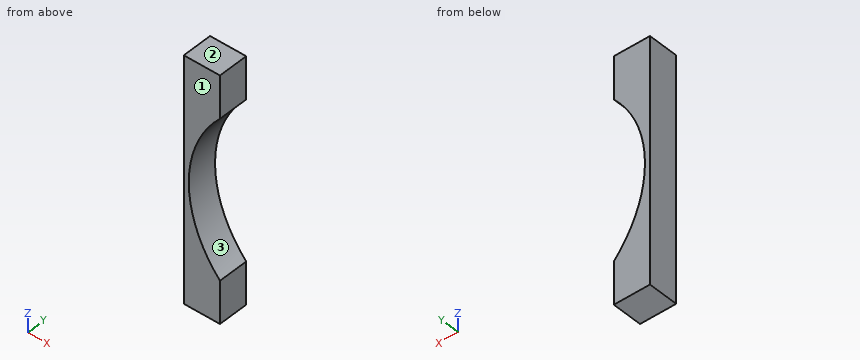
```python
from build123d import *

# Parameters (mm, degrees)
SKETCH1_W           = 24.21
SKETCH1_H           = 6
BOSS_EXTRUDE1_DEPTH = 48.61
CUT_EXTRUDE1_DEPTH  = 53.417790043


with BuildPart() as part:
    # Sketch1 → Boss-Extrude1 (new body)
    with BuildSketch(Plane.XY):
        with Locations((-6.568312856, 6.986625)):
            Rectangle(SKETCH1_W, SKETCH1_H)
    extrude(amount=BOSS_EXTRUDE1_DEPTH)

    # Sketch3 → Cut-Extrude1 (cut, through all)
    with BuildSketch(Plane(origin=(0, 9.986625, 0), x_dir=(1, 0, 0), z_dir=(0, 1, 0))):
        with BuildLine():
            Line((-11.463312856, 0), (-11.463312856, -8.458721642))
            ThreePointArc((-11.463312856, -8.458721642), (-17.673312856, -24.3), (-11.463312856, -40.141278358))
            Line((-11.463312856, -40.141278358), (-11.463312856, -48.61))
            Line((-11.463312856, -48.61), (5.536687144, -48.61))
            Line((5.536687144, -48.61), (5.536687144, 0))
            Line((5.536687144, 0), (-11.463312856, 0))
        make_face()
    extrude(amount=-CUT_EXTRUDE1_DEPTH, mode=Mode.SUBTRACT)


solid = part.part
```
Build history of the part. All positions in model axes, mm. Face numbers are marked on the shaded views. Give positions to 0.01 mm unless a question says otherwise; leave off trailing zeros. Loops run counter-clockwise (first coordinate to the right, second up) from the corner with the lowest first, then second, coordinate; pieces in that order, holes last. Notation, with made-up numbers: (53.25, 2) - (92.25, 2) arc R29 ccw to (92.25, 31) - close; hole circle Ø1 at (23, 48.25). An arc over 180 degrees is marked (long way). Use a Markdown table: item, result.
(1) Band-saw the part on B-B (y = 6.3). Give the cut face in (x, z).
Taken from the geometry:
| item | result |
|---|---|
| outline | (-18.67, 0) - (-11.46, 0) - (-11.46, 8.46) arc R23.31 cw to (-11.46, 40.14) - (-11.46, 48.61) - (-18.67, 48.61) - close |
(2) Band-saw the part on D-D (x = -15.75). Give the cut face in (y, z).
Taken from the geometry:
| item | result |
|---|---|
| outline | (3.99, 0) - (9.99, 0) - (9.99, 15.03) - (3.99, 15.03) - close; (3.99, 33.57) - (9.99, 33.57) - (9.99, 48.61) - (3.99, 48.61) - close |
(3) Band-saw the part on C-C (z = 37.5). Give the cut face in (x, y), and give its area (3 significant figures).
Taken from the geometry:
| item | result |
|---|---|
| outline | (-18.67, 3.99) - (-13.58, 3.99) - (-13.58, 9.99) - (-18.67, 9.99) - close |
| area | 30.6 mm2 |
(4) Pull direction Z, two halves, no side cores. Call the marked faces 1, 2 and 3: +Z half, -Z half, draft (parallel to the pull), parting line (faces both ways), or undercut.
Taken from the geometry:
| item | result |
|---|---|
| face 1 | draft |
| face 2 | +Z half |
| face 3 | undercut |
(5) Band-saw the part on A-A (x = -12). Give the cut face in (y, z).
Taken from the geometry:
| item | result |
|---|---|
| outline | (3.99, 0) - (9.99, 0) - (9.99, 9.06) - (3.99, 9.06) - close; (3.99, 39.54) - (9.99, 39.54) - (9.99, 48.61) - (3.99, 48.61) - close |
(6) Wall check: line 1 along X through (y, z) = (5.45, 25); line 2 along Z through (x, y) = (-11.75, 8.6); line 3 along Z through (x, y) = (-13.5, 5.4). Give the ranges that are in metal, low to high.
Taken from the geometry:
| item | result |
|---|---|
| line 1 | -18.67 to -17.66 |
| line 2 | 0 to 8.77, 39.83 to 48.61 |
| line 3 | 0 to 10.99, 37.61 to 48.61 |
